from build123d import *

# Parameters (mm, degrees)
F1_DEPTH  = 127
F3_DEPTH  = 152.4
F4_W      = 152.4
F4_H      = 25.4
F5_DEPTH  = 50.8
F8_DEPTH  = 25.4
F9_R      = 12.7
F10_R     = 6.35
F11_DEPTH = 50.447222


with BuildPart() as f1:
    # F0 (on Front) → F1 (new body)
    with BuildSketch(Plane.XZ):
        Polygon((0, 50.447222), (0, 0), (38.1, 0), (38.1, 12.7), (114.3, 12.7), (114.3, 0), (152.4, 0), (152.4, 50.447222), align=None)
    extrude(amount=-F1_DEPTH)

    # F2 (on face) → F3 (cut, through all)
    with BuildSketch(Plane.YZ.offset(152.4)):
        Polygon((73.025, 50.447222), (53.975, 50.447222), (53.975, 37.747222), (38.227, 37.747222), (38.227, 25.047222), (89.027, 25.047222), (89.027, 37.747222), (73.025, 37.747222), align=None)
    extrude(amount=-F3_DEPTH, mode=Mode.SUBTRACT)

    # F4 (on face) → F5 (join)
    with BuildSketch(Plane.XY.offset(50.447222)):
        with Locations((76.2, 114.3)):
            Rectangle(F4_W, F4_H)
    extrude(amount=F5_DEPTH)

    # F7 (on face) → F8 (cut, through all)
    with BuildSketch(Plane(origin=(0, 127, 0), x_dir=(-1, 0, 0), z_dir=(0, 1, 0))):
        with BuildLine():
            Line((-76.2, 101.247222), (-114.3, 101.247222))
            ThreePointArc((-114.3, 101.247222), (-76.2, 63.147222), (-38.1, 101.247222))
            Line((-38.1, 101.247222), (-76.2, 101.247222))
        make_face()
    extrude(amount=-F8_DEPTH, mode=Mode.SUBTRACT)

    # F9
    f9_edges = [f1.edges().sort_by_distance(p)[0] for p in [
        (152.4, 114.3, 101.247222),
        (0, 114.3, 101.247222),
    ]]
    fillet(f9_edges, radius=F9_R)

    # F10 (on face) → F11 (cut, through all)
    with BuildSketch(Plane.XY.offset(50.447222)):
        with BuildLine():
            Line((19.05, 19.05), (19.05, 12.7))
            ThreePointArc((19.05, 12.7), (23.540128, 14.559872), (25.4, 19.05))
            ThreePointArc((25.4, 19.05), (19.05, 25.4), (12.7, 19.05))
            Line((12.7, 19.05), (19.05, 19.05))
        make_face()
        with BuildLine():
            ThreePointArc((12.7, 19.05), (14.559872, 14.559872), (19.05, 12.7))
            Line((19.05, 12.7), (19.05, 19.05))
            Line((19.05, 19.05), (12.7, 19.05))
        make_face()
        with Locations((133.35, 19.05)):
            Circle(F10_R)
    extrude(amount=-F11_DEPTH, mode=Mode.SUBTRACT)


solid = f1.part
Verification items for the finished model (mm, model axes). A direction names the side the tool comes from. Coordinates: 2 decimals unless noted, no trailing zeros. Loops run counter-clockwise (first coordinate to the right, second up) from the corner with the lowest first, then second, coordinate; pieces in that order, holes last. Notation, with made-up numbers: (63, -14.5) -> (78, -14.5) arc R9 cw to (78, 1.5) -> close; hole circle Ø10 at (-13, 29.5). An arc over 180 degrees is marked (long way). Answer as a JSON object with one key per item and string values. Group by question number.
Item 1: Sectioned sample at B-B on x = 76.2. Record the boundary of the cut face in (y, z) (3 decimals), plus the area to 3 significant figures.
Item 2: Mould release check, pull along Y, two halves, no side actions. Record for faces 1 (the flat face through (77, 87, 50.447)), 2 (the flat face through (77, 73.025, 44)), 3 (the flat face through (75, 101.6, 59)): +Y half, -Y half, draft (parallel to the pull), parting line (faces both ways), or undercut.
Item 3: Sectioned sample at A-A on x = 133.35. Record the boundary of the cut face in (y, z) (3 decimals).
Item 4: Tool access check on faces 4 (the flat face through (77, 46, 37.747)), 5 (the flat face through (77, 27, 50.447)), 6 (the flat face through (77, 53.975, 44)). Record the directions out of +Z, -Z, +X, -X, +Y, -Y that give a thin tool (end or side, any length) a straight path to the whole face; none if there is none.
Item 5: Depth check by flat-ended pin: pin 1 (23 mm diameter, centred on x = 66.5, y = 49, fed in from -Z); pin 2 (8 mm diameter, centred on y = 61, z = 37.5, fed in from -X); pin 3 (15 mm diameter, centred on x = 56.5, z = 67.5, fed in from -Y); pin 4 (8.5 mm diameter, centred on x = 101, y = 89, fed in from +Z). Enter the tip coordinate at first touch or a pass-through.
Item 6: Scan lines: probe 1 along Y at (x, z) = (133, 27); probe 2 along Z at (x, y) = (130, 77); probe 3 along Y at (x, z) = (50, 42) (3 decimals). Record each from-to range of solid material in increasing order.
Item 7: Sectioned sample at C-C on x = 109. Record the boundary of the cut face in (y, z) (3 decimals), plus the area to 3 significant figures.
Evaluation:
{
 "1": {"outline": "(0, 12.7) -> (127, 12.7) -> (127, 63.147) -> (101.6, 63.147) -> (101.6, 50.447) -> (73.025, 50.447) -> (73.025, 37.747) -> (89.027, 37.747) -> (89.027, 25.047) -> (38.227, 25.047) -> (38.227, 37.747) -> (53.975, 37.747) -> (53.975, 50.447) -> (0, 50.447) -> close", "area": "4,230 mm²"},
 "2": {"face 1": "draft", "face 2": "undercut", "face 3": "-Y half"},
 "3": {"outline": "(0, 0) -> (12.7, 0) -> (12.7, 50.447) -> (0, 50.447) -> close; (25.4, 0) -> (127, 0) -> (127, 101.247) -> (101.6, 101.247) -> (101.6, 50.447) -> (73.025, 50.447) -> (73.025, 37.747) -> (89.027, 37.747) -> (89.027, 25.047) -> (38.227, 25.047) -> (38.227, 37.747) -> (53.975, 37.747) -> (53.975, 50.447) -> (25.4, 50.447) -> close"},
 "4": {"face 4": "+X, -X", "face 5": "+Z, +X, -X, -Y", "face 6": "+Z, +X, -X"},
 "5": {"pin 1": "stops at z = 12.7", "pin 2": "passes through", "pin 3": "stops at y = 101.6", "pin 4": "stops at z = 50.45"},
 "6": {"probe 1": "y = 0 to 12.71, 25.39 to 38.23, 89.03 to 127", "probe 2": "z = 0 to 25.05, 37.75 to 50.45", "probe 3": "y = 0 to 53.975, 73.025 to 127"},
 "7": {"outline": "(0, 12.7) -> (127, 12.7) -> (127, 81.862) -> (101.6, 81.862) -> (101.6, 50.447) -> (73.025, 50.447) -> (73.025, 37.747) -> (89.027, 37.747) -> (89.027, 25.047) -> (38.227, 25.047) -> (38.227, 37.747) -> (53.975, 37.747) -> (53.975, 50.447) -> (0, 50.447) -> close", "area": "4,700 mm²"}
}
